Model file for the job. Use its own axes, mm. Face numbers are marked on the shaded views. A direction names the side the tool comes from. Coordinates: 2 decimals unless noted, no trailing zeros. Loops run counter-clockwise (first coordinate to the right, second up) from the corner with the lowest first, then second, coordinate; pieces in that order, holes last.
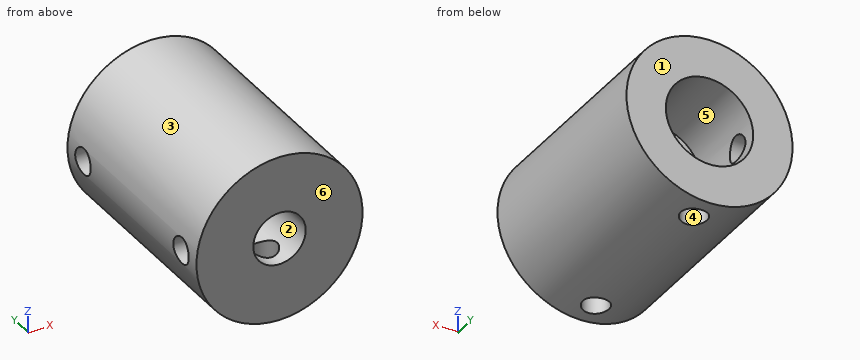
from build123d import *

# Parameters (mm, degrees)
SKETCH_1_R          = 9.5
SKETCH_1_R_2        = 3
EXTRUDE_1_DEPTH     = 25
SKETCH_2_R          = 5
CUT_EXTRUDE_1_DEPTH = 10
SKETCH_3_R          = 1.5
CUT_EXTRUDE_2_DEPTH = 10
SKETCH_4_R          = 1.5
CUT_EXTRUDE_3_DEPTH = 10


with BuildPart() as part:
    # 草图1 → 凸台-拉伸1 (new body)
    with BuildSketch(Plane(origin=(0, 0, 0), x_dir=(1, 0, 0), z_dir=(0, 1, 0))):
        with Locations(Location((0, 0, 0), (0, 0, 270))):
            Circle(SKETCH_1_R)
        with Locations(Location((0, 0, 0), (0, 0, 270))):
            Circle(SKETCH_1_R_2, mode=Mode.SUBTRACT)
    extrude(amount=EXTRUDE_1_DEPTH)

    # 草图2 → 切除-拉伸1 (cut)
    with BuildSketch(Plane(origin=(0, 25, 0), x_dir=(1, 0, 0), z_dir=(0, 1, 0))):
        with Locations(Location((0, 0, 0), (0, 0, 270))):
            Circle(SKETCH_2_R)
    extrude(amount=-CUT_EXTRUDE_1_DEPTH, mode=Mode.SUBTRACT)

    # 草图3 → 切除-拉伸2 (cut)
    with BuildSketch(Plane(origin=(0, 0, 0), x_dir=(0, 0, -1), z_dir=(1, 0, 0))):
        with Locations((0, 3)):
            Circle(SKETCH_3_R)
        with Locations((0, 22)):
            Circle(SKETCH_3_R)
    extrude(amount=-CUT_EXTRUDE_2_DEPTH, mode=Mode.SUBTRACT)

    # 草图4 → 切除-拉伸3 (cut)
    with BuildSketch(Plane.XY):
        with Locations(Location((0, 3, 0), (0, 0, 90))):
            Circle(SKETCH_4_R)
        with Locations((0, 22)):
            Circle(SKETCH_4_R)
    extrude(amount=-CUT_EXTRUDE_3_DEPTH, mode=Mode.SUBTRACT)


solid = part.part
Q1. Flat gauge pins, fed straight in: P1, Ø5, axis at x = 2, z = -5.5, coming from the -Y side; P2, Ø1, axis at y = 6, z = -5, coming from the -X side; P3, Ø2, axis at y = 11.5, z = -5, coming from the +X side; P4, Ø3.5, axis at x = 0, z = 0, coming from the +Y side. Where does each tip first touch, or does it go through?
Answers:
P1: stops at y = 0
P2: stops at x = -8.37
P3: stops at x = 8.62
P4: passes through
Q2. Slice it at A-A (z = 0). List the corners of the cut face in (x, y).
Answers:
outline: (-9.5, 0) - (-3, 0) - (-3, 1.5) - (-9.5, 1.5) - close; (-9.5, 4.5) - (-3, 4.5) - (-3, 15) - (-5, 15) - (-5, 20.5) - (-9.5, 20.5) - close; (-9.5, 23.5) - (-5, 23.5) - (-5, 25) - (-9.5, 25) - close; (3, 0) - (9.5, 0) - (9.5, 25) - (5, 25) - (5, 15) - (3, 15) - close
Q3. Slice it at B-B (x = 0). List the corners of the cut face in (y, z).
Answers:
outline: (0, -9.5) - (1.5, -9.5) - (1.5, -3) - (0, -3) - close; (0, 3) - (15, 3) - (15, 5) - (25, 5) - (25, 9.5) - (0, 9.5) - close; (4.5, -9.5) - (20.5, -9.5) - (20.5, -5) - (15, -5) - (15, -3) - (4.5, -3) - close; (23.5, -9.5) - (25, -9.5) - (25, -5) - (23.5, -5) - close
Q4. Slice it at C-C (y = 22). List the corners of the cut face in (x, z), and give its area (3 significant figures).
Answers:
outline: (-9.38, -1.5) arc R9.5 ccw to (-1.5, -9.38) - (-1.5, -4.77) arc R5 cw to (-4.77, -1.5) - close; (-9.38, 1.5) - (-4.77, 1.5) arc R5 cw (long way) to (1.5, -4.77) - (1.5, -9.38) arc R9.5 ccw (long way) to start
area: 178 mm2
Q5. Drill centre lines: line 1 (Z direction, x = 0, y = 18.5); line 2 (Y direction, x = -7, z = 0.5); line 3 (Y direction, x = -3.25, z = 0). Where is each one in solid material? Low to high.
Answers:
line 1: z = -9.5 to -5, 5 to 9.5
line 2: y = 0 to 1.59, 4.41 to 20.59, 23.41 to 25
line 3: y = 0 to 1.5, 4.5 to 15
Q6. Slice it at D-D (x = -6.5). List the corners of the cut face in (y, z).
Answers:
outline: (0, -6.93) - (25, -6.93) - (25, 6.93) - (0, 6.93) - close; hole circle Ø3 at (3, 0); hole circle Ø3 at (22, 0)
Q7. Which spindle directions (+Z, -Z, +X, -X, +Y, -Y) get a long thin tool onto all of the face, cutting with end or side? Do the marked faces 4, 5 and 6. Say none if no direction does.
Answers:
face 4: -Z
face 5: +Y
face 6: +Z, -Z, +X, -X, -Y
Q8. Mould opens along Z. For the marked faces 1, 2 and 3 say: +Z half, -Z half, draft (parallel to the pull), parting line (faces both ways), or undercut.
Answers:
face 1: draft
face 2: undercut
face 3: parting line
